The model under review builds one solid part; all positions refer to its coordinate system, in mm. A direction names the side the tool comes from. Give positions to 0.01 mm unless a question says otherwise; leave off trailing zeros. Write each loop counter-clockwise with the first axis right and the second up, starting at its lowest first coordinate (ties: lowest second). Pieces come first, ordered by that corner, then holes. Notation, with made-up numbers: (-33.75, -39.75) -> (4.25, -39.75) arc R17 cw to (4.25, -10.75) -> close; hole circle Ø10 at (11, 14.5). An arc over 180 degrees is marked (long way). Use CSV: the item, a comma, the result in double quotes.
```python
from build123d import *

# Parameters (mm, degrees)
SALIENTE_EXTRUIR1_DEPTH = 3
REDONDEO1_R             = 1
REDONDEO2_R             = 0.25


with BuildPart() as part:
    # Croquis1 → Saliente-Extruir1 (new body)
    with BuildSketch(Plane.XY):
        with BuildLine():
            Line((-24, 25), (-24, -25))
            ThreePointArc((-24, -25), (-23.267766953, -26.767766953), (-21.5, -27.5))
            Line((-21.5, -27.5), (-7, -27.5))
            Line((-7, -27.5), (-7, -33.1))
            ThreePointArc((-7, -33.1), (-6.267766953, -34.867766953), (-4.5, -35.6))
            Line((-4.5, -35.6), (8, -35.6))
            Line((8, -35.6), (8, -33.6))
            Line((8, -33.6), (-2, -33.6))
            Line((-2, -33.6), (-2, -30.5))
            Line((-2, -30.5), (8, -30.5))
            Line((8, -30.5), (8, -27.5))
            Line((8, -27.5), (21.5, -27.5))
            ThreePointArc((21.5, -27.5), (23.267766953, -26.767766953), (24, -25))
            Line((24, -25), (24, 25))
            ThreePointArc((24, 25), (23.267766953, 26.767766953), (21.5, 27.5))
            Line((21.5, 27.5), (8, 27.5))
            Line((8, 27.5), (8, 30.5))
            Line((8, 30.5), (-2, 30.5))
            Line((-2, 30.5), (-2, 33.6))
            Line((-2, 33.6), (8, 33.6))
            Line((8, 33.6), (8, 35.6))
            Line((8, 35.6), (-4.5, 35.6))
            ThreePointArc((-4.5, 35.6), (-6.267766953, 34.867766953), (-7, 33.1))
            Line((-7, 33.1), (-7, 27.5))
            Line((-7, 27.5), (-21.5, 27.5))
            ThreePointArc((-21.5, 27.5), (-23.267766953, 26.767766953), (-24, 25))
        make_face()
    extrude(amount=SALIENTE_EXTRUIR1_DEPTH)

    # Redondeo1
    redondeo1_edges = [part.edges().sort_by_distance(p)[0] for p in [
        (-7, 27.5, 1.5),
        (8, 35.6, 1.5),
        (8, 27.5, 1.5),
        (8, -27.5, 1.5),
        (8, -35.6, 1.5),
        (-7, -27.5, 1.5),
    ]]
    fillet(redondeo1_edges, radius=REDONDEO1_R)

    # Redondeo2
    redondeo2_edges = [part.edges().sort_by_distance(p)[0] for p in [
        (8, 33.6, 1.5),
        (-2, 33.6, 1.5),
        (-2, 30.5, 1.5),
        (8, 30.5, 1.5),
        (8, -30.5, 1.5),
        (-2, -30.5, 1.5),
        (-2, -33.6, 1.5),
        (8, -33.6, 1.5),
    ]]
    fillet(redondeo2_edges, radius=REDONDEO2_R)


solid = part.part
```
Q1. Machinability: for faces 1 (the flat face through (8, 29, 1)), 2 (the flat face through (-7, -31, 1)), 3 (the flat face through (-15, 27.5, 1)), 4 (the flat face through (3, -30.5, 1)), which of the approach directions +Z, -Z, +X, -X, +Y, -Y give a long, thin tool a straight path to every point of the face, cutting with its end or side? Answer none if there is none.
Derived:
face 1,"+Z, -Z, +X, +Y"
face 2,"+Z, -Z, -X, -Y"
face 3,"+Z, -Z, -X, +Y"
face 4,"+Z, -Z, +X"
Q2. Consider section A-A (x = 5.5). Write out the cut boundary in (y, z).
Derived:
outline,"(-35.6, 0) -> (-33.6, 0) -> (-33.6, 3) -> (-35.6, 3) -> close; (-30.5, 0) -> (30.5, 0) -> (30.5, 3) -> (-30.5, 3) -> close; (33.6, 0) -> (35.6, 0) -> (35.6, 3) -> (33.6, 3) -> close"
Q3. To check wall thickness, follow probe 1 along Y at (x, z) = (5.5, 0.7); probe 2 along X at (y, z) = (-32, 1); probe 3 along Y at (x, z) = (10.5, 2.1). State the ranges of each line that lie inside material, in increasing order.
Derived:
probe 1,"y = -35.6 to -33.6, -30.5 to 30.5, 33.6 to 35.6"
probe 2,"x = -7 to -2"
probe 3,"y = -27.5 to 27.5"
Q4. Insertion check: pin 1 (1.3 mm diameter, centred on y = 32, z = 1, fed in from +X); pin 2 (1.5 mm diameter, centred on x = -17.5, z = 1.5, fed in from -Y); pin 3 (3 mm diameter, centred on x = 13.5, y = -12, fed in from -Z); pin 4 (1.5 mm diameter, centred on x = 12.5, z = 1.5, fed in from +Y). Each pin has a flat end and moves straight along its axis. Give the tip position at first contact, or say it passes through.
Derived:
pin 1,"stops at x = -2"
pin 2,"stops at y = -27.5"
pin 3,"stops at z = 0"
pin 4,"stops at y = 27.5"
Q5. Consider section B-B (x = 19). Write out the cut boundary in (y, z), then the cut area to 3 significant figures.
Derived:
outline,"(-27.5, 0) -> (27.5, 0) -> (27.5, 3) -> (-27.5, 3) -> close"
area,"165 mm2"
